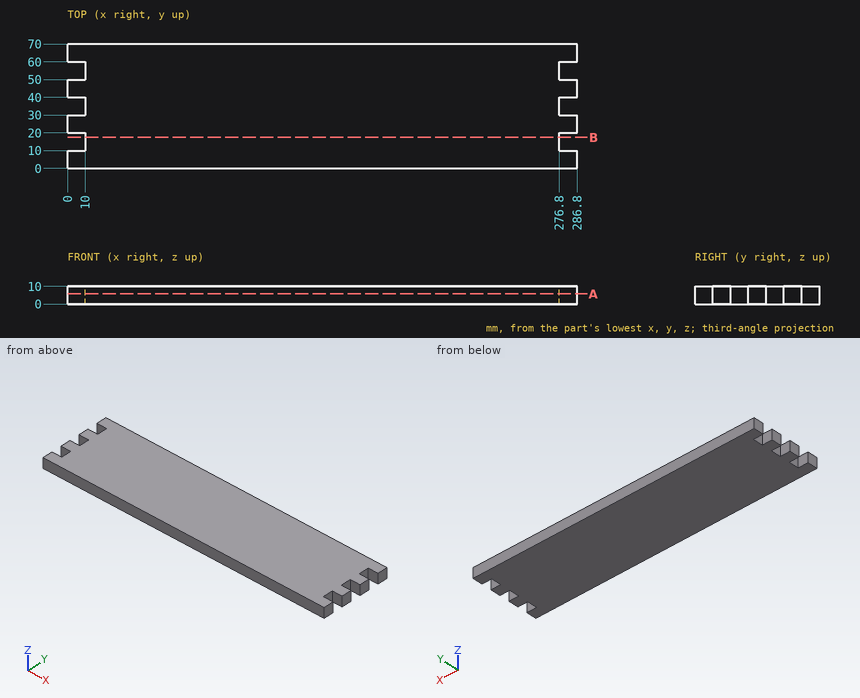
For this review, use the dimensioned drawing (mm, ordinates from the lowest corner) and the shaded views. Round coordinates to 2 decimals unless told otherwise and drop trailing zeros. Order: outer loops, then holes, each group sorted by start corner. A loop starts at its lowest first (then second) coordinate and runs counter-clockwise, first axis right, second up. Notation, with made-up numbers: M -29.75,-18.75 L 7.25,-18.75 A20 cw 7.25,-14.75 Z; hole C -17.5,60 d2. An arc over 180 degrees is marked long. Use a Markdown table: item, result. Add a question column.
Item 1: Insertion check: pin 1 (3 mm diameter, centred on y = 54.5, z = 6.5, fed in from +X); pin 2 (5 mm diameter, centred on x = 3.5, z = 4, fed in from -Y); pin 3 (3 mm diameter, centred on y = 35.5, z = 7.5, fed in from -X). Each pin has a flat end and moves straight along its axis. Give the tip position at first contact, or say it passes through.
Item 2: Add section A-A, the plane z = 5.75. Give the boundary of the cut face in (x, y).
Item 3: Add section B-B, the plane y = 17.5. Give the boundary of the cut face in (x, z), then the cut area to 3 significant figures.
Item 4: To check wall thickness, follow line 1 along X through (y, z) = (19, 1). State the ranges of the line that lie inside material, in increasing order.
Geometry results:
| question | item | result |
|---|---|---|
| 1 | pin 1 | stops at x = 276.8 |
| 1 | pin 2 | stops at y = 0 |
| 1 | pin 3 | stops at x = 10 |
| 2 | outline | M 0,0 L 286.8,0 L 286.8,10 L 276.8,10 L 276.8,20 L 286.8,20 L 286.8,30 L 276.8,30 L 276.8,40 L 286.8,40 L 286.8,50 L 276.8,50 L 276.8,60 L 286.8,60 L 286.8,70 L 0,70 L 0,60 L 10,60 L 10,50 L 0,50 L 0,40 L 10,40 L 10,30 L 0,30 L 0,20 L 10,20 L 10,10 L 0,10 Z |
| 3 | outline | M 10,0 L 276.8,0 L 276.8,10 L 10,10 Z |
| 3 | area | 2,670 mm² |
| 4 | line 1 | x = 10 to 276.8 |
